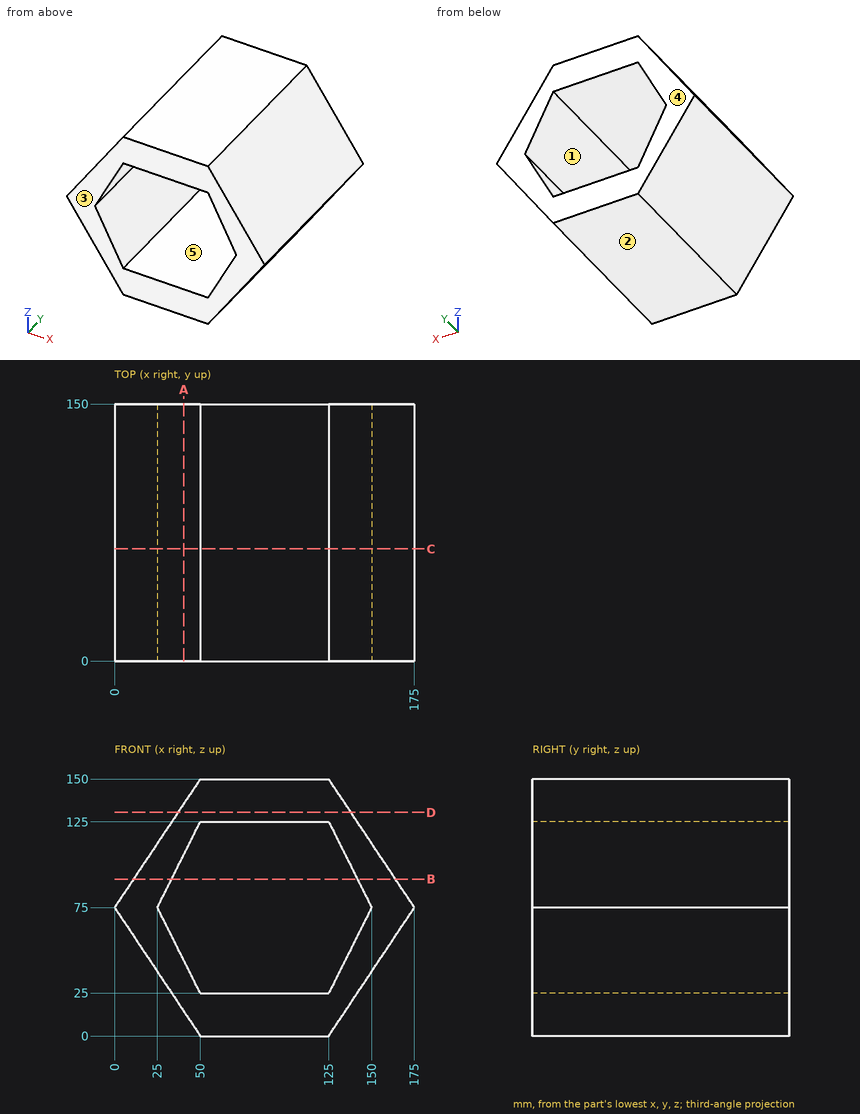
Drawing for the job (mm, zero at the part's lowest x, y, z). A direction names the side the tool comes from. Round coordinates to 2 decimals unless told otherwise and drop trailing zeros. Order: outer loops, then holes, each group sorted by start corner. A loop starts at its lowest first (then second) coordinate and runs counter-clockwise, first axis right, second up.
Item 1: Saw through at A-A on x = 40.5. Write the cut outline in (y, z).
Item 2: Saw through at C-C on y = 65.5. Write the cut outline in (x, z).
Item 3: Saw through at D-D on z = 130.5. Write the cut outline in (x, y).
Item 4: Tool access for the marked faces 4 and 5: list every direction of +Z, -Z, +X, -X, +Y, -Y with a clear straight run to the whole face (end or side of a thin tool).
Item 5: Pin check, flat tips, straight feed: pin 1 (10 mm diameter, centred on x = 32.5, y = 89.5, fed in from +Z); pin 2 (2 mm diameter, centred on y = 20.5, z = 134.5, fed in from +X); pin 3 (6 mm diameter, centred on y = 41.5, z = 110.5, fed in from -X). Stop position of each tip, or through.
Item 6: Mould opens along Z. For the marked faces 1, 2 and 3 say: pulls with the +Z half, pulls with the -Z half, needs draft (parallel to the pull), parting line crosses it, or undercut.
Item 7: Probe line 1 along Z through (x, y) = (70, 29); line 2 along Z through (x, y) = (146, 37.5); line 3 along X through (y, z) = (114, 33.5). List the from-to ranges inside material, lowest first.
Item 8: Saw through at B-B on z = 91.5. Write the cut outline in (x, y), then the cut area to 4 significant figures.
Reported:
1. outline: (0, 14.25) - (150, 14.25) - (150, 44) - (0, 44) - close; (0, 106) - (150, 106) - (150, 135.75) - (0, 135.75) - close
2. outline: (0, 75) - (50, 0) - (125, 0) - (175, 75) - (125, 150) - (50, 150) - close; hole (25, 75) - (50, 25) - (125, 25) - (150, 75) - (125, 125) - (50, 125) - close
3. outline: (37, 0) - (138, 0) - (138, 150) - (37, 150) - close
4. face 4: +Z, -Z, +X, -X, +Y
4. face 5: +Y, -Y
5. pin 1: stops at z = 131.25
5. pin 2: stops at x = 136
5. pin 3: stops at x = 21.67
6. face 1: undercut
6. face 2: pulls with the -Z half
6. face 3: needs draft
7. line 1: z = 0 to 25, 125 to 150
7. line 2: z = 31.5 to 67, 83 to 118.5
7. line 3: x = 27.67 to 45.75, 129.25 to 147.33
8. outline: (11, 0) - (33.25, 0) - (33.25, 150) - (11, 150) - close; (141.75, 0) - (164, 0) - (164, 150) - (141.75, 150) - close
8. area: 6,675 mm2
